For this review, take the finished solid that the model builds, in its own axes (mm). Face numbers are marked on the shaded views. A direction names the side the tool comes from. Round coordinates to 2 decimals unless told otherwise and drop trailing zeros. Loops run counter-clockwise (first coordinate to the right, second up) from the corner with the lowest first, then second, coordinate; pieces in that order, holes last.
1) Tool access review of the marked faces 4, 5, 6, 7 and 8: name each direction out of +Z, -Z, +X, -X, +Y, -Y from which nothing blocks a thin tool from reaching the whole face with its end or side.
2) Take a section at B-B (x = -52). State the section outline as (y, z) points.
3) Take a section at A-A (x = 0). State the section outline as (y, z) points (3 decimals).
4) Mouldability with a two-part tool opening along X and no side actions: class the marked faces 1, 2 and 3 as pulls with the +X half, pulls with the -X half, needs draft (parallel to the pull), parting line crosses it, or undercut.
5) Take a section at C-C (y = 5). Give the number of separate pieces and of enclosed holes in the cut face, then the cut area to 3 significant figures.
6) Insertion check: pin 1 (1 mm diameter, centred on y = -13.5, z = 3.5, fed in from -X); pin 2 (3 mm diameter, centred on y = -2.5, z = 6, fed in from +X); pin 3 (3 mm diameter, centred on x = -59.5, z = 10.5, fed in from +Y). Each pin has a flat end and moves straight along its axis. Give the tip position at first contact, or say it passes through.
7) Wall thickness on L1, parallel to X at y = 4.5, z = 10.5; L2, parallel to X at y = -7.5, z = 11.75; L3, parallel to Y at x = -10.5, z = 7: over which ranges is each line inside the solid? List them lowest first.
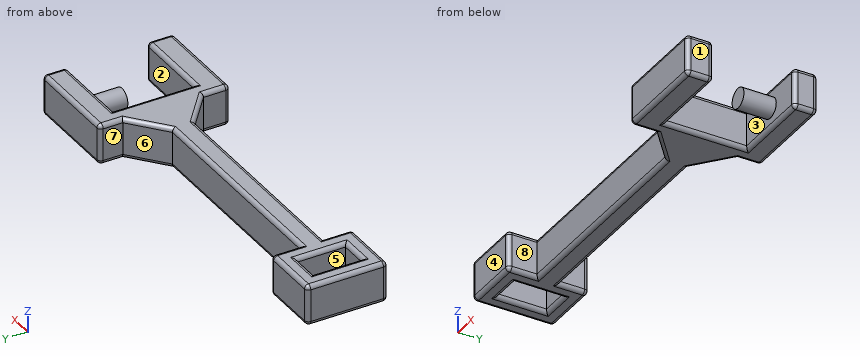
```python
from build123d import *

# Parameters (mm, degrees)
F0_W     = 8.89
F0_H     = 15.24
F1_DEPTH = 12.7
F2_R     = 3.175
F5_DEPTH = 10.16
F6_R     = 1.27


# Not quite as in the source:
# - the program builds the solid bodies; features that only make, move or delete a surface that nothing else refers to are left out


with BuildPart() as f1:
    # F0 (on Top) → F1 (new body)
    with BuildSketch(Plane.XY):
        Polygon((-12.7, 12.7), (12.7, 12.7), (12.7, 20.1094653457), (-17.78, 20.1094653457), (-17.78, 12.7), (-28.8291541207, 3.5404531619), (-97.5522994995, 3.5404531619), (-97.5522994995, 12.7), (-116.6022994995, 12.7), (-116.6022994995, -12.7), (-97.5522994995, -12.7), (-97.5522994995, -3.5404531619), (-28.8291541207, -3.5404531619), (-17.78, -12.7), (-17.78, -20.9651887417), (12.7, -20.9651887417), (12.7, -12.7), (-12.7, -12.7), align=None)
        with Locations((-107.0772994995, 0)):
            Rectangle(F0_W, F0_H, mode=Mode.SUBTRACT)
    extrude(amount=F1_DEPTH)

    # F2 (on face) → F5 (join)
    with BuildSketch(Plane.XZ.offset(-12.7)):
        with Locations((0, 6.35)):
            Circle(F2_R)
    extrude(amount=F5_DEPTH)

    # F6
    f6_edges = [f1.edges().sort_by_distance(p)[0] for p in [
        (-63.190727, -3.540453, 12.7),
        (-63.190727, 3.540453, 12.7),
        (-63.190727, -3.540453, 0),
        (-107.077299, -12.7, 12.7),
        (-97.552299, -8.120227, 12.7),
        (-97.552299, -12.7, 6.35),
        (-97.552299, -8.120227, 0),
        (-107.077299, -12.7, 0),
        (-116.602299, -12.7, 6.35),
        (-116.602299, 0, 12.7),
        (-107.077299, 12.7, 12.7),
        (-97.552299, 8.120227, 12.7),
        (-102.632299, 0, 12.7),
        (-107.077299, 7.62, 12.7),
        (-111.522299, 0, 12.7),
        (-107.077299, -7.62, 12.7),
        (-116.602299, 12.7, 6.35),
        (-116.602299, 0, 0),
        (-111.522299, 0, 0),
        (-107.077299, 7.62, 0),
        (-102.632299, 0, 0),
        (-107.077299, -7.62, 0),
        (-107.077299, 12.7, 0),
        (-97.552299, 12.7, 6.35),
        (-97.552299, 8.120227, 0),
        (-63.190727, 3.540453, 0),
        (-17.78, 20.109465, 6.35),
        (-23.304577, 8.120227, 12.7),
        (-23.304577, 8.120227, 0),
        (-17.78, 16.404733, 0),
        (-17.78, 16.404733, 12.7),
        (-2.54, 20.109465, 12.7),
        (-2.54, 20.109465, 0),
        (0, 12.7, 0),
        (12.7, 16.404733, 0),
        (12.7, 20.109465, 6.35),
        (12.7, -12.7, 6.35),
        (0, -12.7, 0),
        (12.7, -16.832594, 0),
        (-2.54, -20.965189, 0),
        (-17.78, -16.832594, 0),
        (-12.7, 0, 0),
        (-23.304577, -8.120227, 0),
        (-23.304577, -8.120227, 12.7),
        (-12.7, 0, 12.7),
        (0, 12.7, 12.7),
        (12.7, 16.404733, 12.7),
        (12.7, 12.7, 6.35),
        (-17.78, -16.832594, 12.7),
        (-17.78, -20.965189, 6.35),
        (-2.54, -20.965189, 12.7),
        (0, -12.7, 12.7),
        (12.7, -16.832594, 12.7),
        (12.7, -20.965189, 6.35),
    ]]
    fillet(f6_edges, radius=F6_R)


solid = f1.part
```
Response:
1. face 4: +Z, -Z, -X, -Y
1. face 5: +Z, -Z
1. face 6: +Z, -Z, +Y
1. face 7: +Z, -Z, -X, +Y
1. face 8: +Z, -Z, -Y
2. outline: (-3.54, 1.27) arc R1.27 ccw to (-2.27, 0) - (2.27, 0) arc R1.27 ccw to (3.54, 1.27) - (3.54, 11.43) arc R1.27 ccw to (2.27, 12.7) - (-2.27, 12.7) arc R1.27 ccw to (-3.54, 11.43) - close
3. outline: (-20.965, 1.27) arc R1.27 ccw to (-19.695, 0) - (-13.97, 0) arc R1.27 ccw to (-12.7, 1.27) - (-12.7, 11.43) arc R1.27 ccw to (-13.97, 12.7) - (-19.695, 12.7) arc R1.27 ccw to (-20.965, 11.43) - close; (2.54, 3.175) - (12.7, 3.175) - (12.7, 1.27) arc R1.27 ccw to (13.97, 0) - (18.839, 0) arc R1.27 ccw to (20.109, 1.27) - (20.109, 11.43) arc R1.27 ccw to (18.839, 12.7) - (13.97, 12.7) arc R1.27 ccw to (12.7, 11.43) - (12.7, 9.525) - (2.54, 9.525) - close
4. face 1: pulls with the +X half
4. face 2: needs draft
4. face 3: undercut
5. separate pieces: 4
5. enclosed holes: 0
5. area: 339 mm2
6. pin 1: stops at x = -17.78
6. pin 2: stops at x = -12.7
6. pin 3: stops at y = 3.54
7. L1: x = -116.6 to -111.52, -102.63 to -97.55, -27.67 to -12.7
7. L2: x = -116.56 to -111.56, -102.59 to -97.59, -23.99 to -12.74
7. L3: y = -20.97 to -12.7, 12.7 to 20.11
